Check sheet for the modelled part. Datum: model origin and axes. Units: mm. Round coordinates to 2 decimals unless told otherwise and drop trailing zeros. Write each loop counter-clockwise with the first axis right and the second up, starting at its lowest first coordinate (ties: lowest second). Pieces come first, ordered by that corner, then holes.
Item 1: Go/stop test with flat-tipped pins: pin 1 Ø1.8 at (x, z) = (274.26, -16.26) entering from -Y; pin 2 Ø1 at (x, y) = (102.5, 2) entering from -Z; pin 3 Ø1 at (y, z) = (1, -34.5) entering from -X; pin 4 Ø1 at (x, y) = (-4, 0.5) entering from -Z. Record where each tip stops, or that it passes through.
Item 2: Cross-section at B-B on x = -23.5. Enter the section's corners in (y, z), plus the area to 3 significant figures.
Item 3: Cross-section at C-C on y = 1.1. Count the separate pieces of the cut face and the enclosed holes in it, plus the area to 3 significant figures.
Item 4: Cross-section at A-A on x = 235. Enter the section's corners in (y, z), plus the area to 3 significant figures.
Item 5: Material ranges on line 1 (X direction, y = 0.65, z = -28); line 2 (X direction, y = 1, z = 19.5); line 3 (Z direction, x = -20, y = 1.25), recorded low to high.
from build123d import *

# Parameters (mm, degrees)
SKETCH_1_R               = 1.5
SKETCH_1_R_2             = 37.5
SKETCH_1_R_3             = 9
SKETCH_1_R_4             = 2
EXTRUDE_1_DEPTH          = 3
SKETCH_2_R               = 1.25
CUT_EXTRUDE_1_DEPTH      = 10
CUT_EXTRUDE_2_DEPTH      = 10
CUT_EXTRUDE_3_DEPTH      = 287.481238478
CUT_EXTRUDE_3_DEPTH_BACK = 287.481238478
SKETCH_4_R               = 1.5


with BuildPart() as part:
    # 草图1 → 凸台-拉伸1 (new body)
    with BuildSketch(Plane(origin=(0, 0, 0), x_dir=(1, 0, 0), z_dir=(0, 1, 0))):
        with BuildLine():
            Line((71.271215686, 30), (163.728784314, 30))
            ThreePointArc((163.728784314, 30), (189.096168452, 33.068787794), (213, 42.09809972))
            ThreePointArc((213, 42.09809972), (282.5, 0), (213, -42.09809972))
            ThreePointArc((213, -42.09809972), (189.096168452, -33.068787794), (163.728784314, -30))
            Line((163.728784314, -30), (71.271215686, -30))
            ThreePointArc((71.271215686, -30), (45.903831548, -33.068787794), (22, -42.09809972))
            ThreePointArc((22, -42.09809972), (-47.5, 0), (22, 42.09809972))
            ThreePointArc((22, 42.09809972), (45.903831548, 33.068787794), (71.271215686, 30))
        make_face()
        with Locations(Location((218.735954124, 39.264880132, 0), (0, 0, 270))):
            Circle(SKETCH_1_R, mode=Mode.SUBTRACT)
        with Locations(Location((251.264045876, 39.264880132, 0), (0, 0, 270))):
            Circle(SKETCH_1_R, mode=Mode.SUBTRACT)
        with Locations(Location((274.264880132, 16.264045876, 0), (0, 0, 270))):
            Circle(SKETCH_1_R, mode=Mode.SUBTRACT)
        with Locations(Location((274.264880132, -16.264045876, 0), (0, 0, 270))):
            Circle(SKETCH_1_R, mode=Mode.SUBTRACT)
        with Locations(Location((251.264045876, -39.264880132, 0), (0, 0, 270))):
            Circle(SKETCH_1_R, mode=Mode.SUBTRACT)
        with Locations(Location((218.735954124, -39.264880132, 0), (0, 0, 270))):
            Circle(SKETCH_1_R, mode=Mode.SUBTRACT)
        with Locations(Location((195.735119868, -16.264045876, 0), (0, 0, 270))):
            Circle(SKETCH_1_R, mode=Mode.SUBTRACT)
        with Locations(Location((195.735119868, 16.264045876, 0), (0, 0, 270))):
            Circle(SKETCH_1_R, mode=Mode.SUBTRACT)
        with Locations(Location((235, 0, 0), (0, 0, 270))):
            Circle(SKETCH_1_R_2, mode=Mode.SUBTRACT)
        with Locations(Location((-16.264045876, 39.264880132, 0), (0, 0, 270))):
            Circle(SKETCH_1_R, mode=Mode.SUBTRACT)
        with Locations(Location((16.264045876, 39.264880132, 0), (0, 0, 270))):
            Circle(SKETCH_1_R, mode=Mode.SUBTRACT)
        with Locations(Location((39.264880132, 16.264045876, 0), (0, 0, 270))):
            Circle(SKETCH_1_R, mode=Mode.SUBTRACT)
        with Locations(Location((39.264880132, -16.264045876, 0), (0, 0, 270))):
            Circle(SKETCH_1_R, mode=Mode.SUBTRACT)
        with Locations(Location((16.264045876, -39.264880132, 0), (0, 0, 270))):
            Circle(SKETCH_1_R, mode=Mode.SUBTRACT)
        with Locations(Location((-16.264045876, -39.264880132, 0), (0, 0, 270))):
            Circle(SKETCH_1_R, mode=Mode.SUBTRACT)
        with Locations(Location((-39.264880132, -16.264045876, 0), (0, 0, 270))):
            Circle(SKETCH_1_R, mode=Mode.SUBTRACT)
        with Locations(Location((-39.264880132, 16.264045876, 0), (0, 0, 270))):
            Circle(SKETCH_1_R, mode=Mode.SUBTRACT)
        with Locations(Location((0, 0, 0), (0, 0, 270))):
            Circle(SKETCH_1_R_3, mode=Mode.SUBTRACT)
        with Locations(Location((-6.783865663, 11.75, 0), (0, 0, 270))):
            Circle(SKETCH_1_R, mode=Mode.SUBTRACT)
        with Locations(Location((6.783865663, 11.75, 0), (0, 0, 270))):
            Circle(SKETCH_1_R, mode=Mode.SUBTRACT)
        with Locations(Location((13.567731326, 0, 0), (0, 0, 270))):
            Circle(SKETCH_1_R, mode=Mode.SUBTRACT)
        with Locations(Location((6.783865663, -11.75, 0), (0, 0, 270))):
            Circle(SKETCH_1_R, mode=Mode.SUBTRACT)
        with Locations(Location((-6.783865663, -11.75, 0), (0, 0, 270))):
            Circle(SKETCH_1_R, mode=Mode.SUBTRACT)
        with Locations(Location((-13.567731326, 0, 0), (0, 0, 270))):
            Circle(SKETCH_1_R, mode=Mode.SUBTRACT)
        with Locations(Location((0, 13.856406461, 0), (0, 0, 270))):
            Circle(SKETCH_1_R_4, mode=Mode.SUBTRACT)
        with Locations(Location((-12, -6.92820323, 0), (0, 0, 270))):
            Circle(SKETCH_1_R_4, mode=Mode.SUBTRACT)
        with Locations(Location((12, -6.92820323, 0), (0, 0, 270))):
            Circle(SKETCH_1_R_4, mode=Mode.SUBTRACT)
    extrude(amount=EXTRUDE_1_DEPTH)

    # 草图2 → 切除-拉伸1 (cut)
    with BuildSketch(Plane.XZ):
        with Locations(Location((190.288457303, 28.213023457, 0), (0, 0, 270))):
            Circle(SKETCH_2_R)
        with Locations(Location((141.728784314, 25, 0), (0, 0, 270))):
            Circle(SKETCH_2_R)
        with Locations(Location((93.271215686, 25, 0), (0, 0, 270))):
            Circle(SKETCH_2_R)
        with Locations(Location((44.711542697, 28.213023457, 0), (0, 0, 270))):
            Circle(SKETCH_2_R)
        with Locations(Location((44.711542697, -28.213023457, 0), (0, 0, 270))):
            Circle(SKETCH_2_R)
        with Locations(Location((93.271215686, -25, 0), (0, 0, 270))):
            Circle(SKETCH_2_R)
        with Locations(Location((141.728784314, -25, 0), (0, 0, 270))):
            Circle(SKETCH_2_R)
        with Locations(Location((190.288457303, -28.213023457, 0), (0, 0, 270.000000002))):
            Circle(SKETCH_2_R)
    extrude(amount=-CUT_EXTRUDE_1_DEPTH, mode=Mode.SUBTRACT)

    # 草图3 → 切除-拉伸2 (cut)
    with BuildSketch(Plane.XZ):
        with BuildLine():
            Line((3.494651309, 34.205809627), (1.886243278, 21.988737715))
            ThreePointArc((1.886243278, 21.988737715), (2.52132569, 19.251580515), (4.799973695, 17.607462978))
            ThreePointArc((4.799973695, 17.607462978), (9.125, 15.804963619), (12.848523388, 12.960630646))
            ThreePointArc((12.848523388, 12.960630646), (15.411694944, 11.809322357), (18.099683819, 12.627903454))
            Line((18.099683819, 12.627903454), (27.875774439, 20.129361624))
            ThreePointArc((27.875774439, 20.129361624), (29.425472637, 22.953753578), (28.390378431, 26.004545998))
            ThreePointArc((28.390378431, 26.004545998), (19.25, 33.341978046), (8.325408233, 37.589061943))
            ThreePointArc((8.325408233, 37.589061943), (5.165797392, 36.960083611), (3.494651309, 34.205809627))
        make_face()
        with BuildLine():
            Line((31.370425748, 14.076448003), (19.985927097, 9.360834261))
            ThreePointArc((19.985927097, 9.360834261), (17.933020634, 7.442258159), (17.648497083, 4.646832332))
            ThreePointArc((17.648497083, 4.646832332), (18.25, 0), (17.648497083, -4.646832332))
            ThreePointArc((17.648497083, -4.646832332), (17.933020634, -7.442258159), (19.985927097, -9.360834261))
            Line((19.985927097, -9.360834261), (31.370425748, -14.076448003))
            ThreePointArc((31.370425748, -14.076448003), (34.591270029, -14.006330033), (36.715786664, -11.584515945))
            ThreePointArc((36.715786664, -11.584515945), (38.5, 0), (36.715786664, 11.584515945))
            ThreePointArc((36.715786664, 11.584515945), (34.591270029, 14.006330033), (31.370425748, 14.076448003))
        make_face()
        with BuildLine():
            Line((27.875774439, -20.129361624), (18.099683819, -12.627903454))
            ThreePointArc((18.099683819, -12.627903454), (15.411694944, -11.809322357), (12.848523388, -12.960630646))
            ThreePointArc((12.848523388, -12.960630646), (9.125, -15.804963619), (4.799973695, -17.607462978))
            ThreePointArc((4.799973695, -17.607462978), (2.52132569, -19.251580515), (1.886243278, -21.988737715))
            Line((1.886243278, -21.988737715), (3.494651309, -34.205809627))
            ThreePointArc((3.494651309, -34.205809627), (5.165797392, -36.960083611), (8.325408233, -37.589061943))
            ThreePointArc((8.325408233, -37.589061943), (19.25, -33.341978046), (28.390378431, -26.004545998))
            ThreePointArc((28.390378431, -26.004545998), (29.425472637, -22.953753578), (27.875774439, -20.129361624))
        make_face()
        with BuildLine():
            Line((-3.494651309, -34.205809627), (-1.886243278, -21.988737715))
            ThreePointArc((-1.886243278, -21.988737715), (-2.52132569, -19.251580515), (-4.799973695, -17.607462978))
            ThreePointArc((-4.799973695, -17.607462978), (-9.125, -15.804963619), (-12.848523388, -12.960630646))
            ThreePointArc((-12.848523388, -12.960630646), (-15.411694944, -11.809322357), (-18.099683819, -12.627903454))
            Line((-18.099683819, -12.627903454), (-27.875774439, -20.129361624))
            ThreePointArc((-27.875774439, -20.129361624), (-29.425472637, -22.953753578), (-28.390378431, -26.004545998))
            ThreePointArc((-28.390378431, -26.004545998), (-19.25, -33.341978046), (-8.325408233, -37.589061943))
            ThreePointArc((-8.325408233, -37.589061943), (-5.165797392, -36.960083611), (-3.494651309, -34.205809627))
        make_face()
        with BuildLine():
            Line((-31.370425748, -14.076448003), (-19.985927097, -9.360834261))
            ThreePointArc((-19.985927097, -9.360834261), (-17.933020634, -7.442258159), (-17.648497083, -4.646832332))
            ThreePointArc((-17.648497083, -4.646832332), (-18.25, 0), (-17.648497083, 4.646832332))
            ThreePointArc((-17.648497083, 4.646832332), (-17.933020634, 7.442258159), (-19.985927097, 9.360834261))
            Line((-19.985927097, 9.360834261), (-31.370425748, 14.076448003))
            ThreePointArc((-31.370425748, 14.076448003), (-34.591270029, 14.006330033), (-36.715786664, 11.584515945))
            ThreePointArc((-36.715786664, 11.584515945), (-38.5, 0), (-36.715786664, -11.584515945))
            ThreePointArc((-36.715786664, -11.584515945), (-34.591270029, -14.006330033), (-31.370425748, -14.076448003))
        make_face()
        with BuildLine():
            Line((-27.875774439, 20.129361624), (-18.099683819, 12.627903454))
            ThreePointArc((-18.099683819, 12.627903454), (-15.411694944, 11.809322357), (-12.848523388, 12.960630646))
            ThreePointArc((-12.848523388, 12.960630646), (-9.125, 15.804963619), (-4.799973695, 17.607462978))
            ThreePointArc((-4.799973695, 17.607462978), (-2.52132569, 19.251580515), (-1.886243278, 21.988737715))
            Line((-1.886243278, 21.988737715), (-3.494651309, 34.205809627))
            ThreePointArc((-3.494651309, 34.205809627), (-5.165797392, 36.960083611), (-8.325408233, 37.589061943))
            ThreePointArc((-8.325408233, 37.589061943), (-19.25, 33.341978046), (-28.390378431, 26.004545998))
            ThreePointArc((-28.390378431, 26.004545998), (-29.425472637, 22.953753578), (-27.875774439, 20.129361624))
        make_face()
    extrude(amount=-CUT_EXTRUDE_2_DEPTH, mode=Mode.SUBTRACT)

    # 草图4 → 切除-拉伸3 (cut, two sides: drawn at the far end of the back side and taken through both)
    with BuildSketch(Plane(origin=(0, 3, 0), x_dir=(1, 0, 0), z_dir=(0, 1, 0)).offset(-CUT_EXTRUDE_3_DEPTH_BACK)):
        with Locations(Location((68.264880132, -16.264045876, 0), (0, 0, 270))):
            Circle(SKETCH_4_R)
        with Locations(Location((110.264880132, -16.264045876, 0), (0, 0, 270))):
            Circle(SKETCH_4_R)
        with Locations(Location((181.264880132, -16.264045876, 0), (0, 0, 270))):
            Circle(SKETCH_4_R)
        with Locations(Location((152.264880132, -16.264045876, 0), (0, 0, 270))):
            Circle(SKETCH_4_R)
        with Locations(Location((181.264880132, 16.264045876, 0), (0, 0, 270))):
            Circle(SKETCH_4_R)
        with Locations(Location((152.264880132, 16.264045876, 0), (0, 0, 270))):
            Circle(SKETCH_4_R)
        with Locations(Location((110.264880132, 16.264045876, 0), (0, 0, 270))):
            Circle(SKETCH_4_R)
        with Locations(Location((68.264880132, 16.264045876, 0), (0, 0, 270))):
            Circle(SKETCH_4_R)
    extrude(amount=CUT_EXTRUDE_3_DEPTH + CUT_EXTRUDE_3_DEPTH_BACK, mode=Mode.SUBTRACT)


solid = part.part
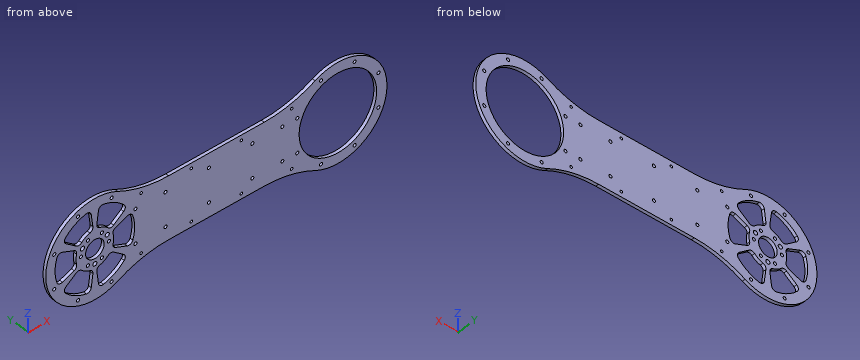
Response values:
1. pin 1: passes through
1. pin 2: stops at z = -30
1. pin 3: stops at x = -33.17
1. pin 4: stops at z = -47.37
2. outline: (0, -41.28) - (3, -41.28) - (3, -30.5) - (0, -30.5) - close; (0, -16.77) - (3, -16.77) - (3, -10.82) - (0, -10.82) - close; (0, 10.82) - (3, 10.82) - (3, 16.77) - (0, 16.77) - close; (0, 30.5) - (3, 30.5) - (3, 41.28) - (0, 41.28) - close
2. area: 100 mm2
3. separate pieces: 1
3. enclosed holes: 49
3. area: 15,500 mm2
4. outline: (0, -47.5) - (3, -47.5) - (3, -37.5) - (0, -37.5) - close; (0, 37.5) - (3, 37.5) - (3, 47.5) - (0, 47.5) - close
4. area: 60.0 mm2
5. line 1: x = -38.37 to -26.42, -2.68 to 2.68, 26.42 to 43.48, 45.94 to 189.06, 191.52 to 210.06, 259.94 to 273.37
5. line 2: x = -43.31 to -27.06, -2.37 to 2.37, 27.06 to 202.97, 267.03 to 278.31
5. line 3: z = -43.08 to -32.9, -14.09 to -9.37, 9.37 to 14.09, 32.9 to 43.08
